Part print with two shaded views. Sizes in mm from the minimum x, y, z corner. Round coordinates to 2 decimals unless told otherwise and drop trailing zeros. Loops run counter-clockwise (first coordinate to the right, second up) from the corner with the lowest first, then second, coordinate; pieces in that order, holes last. Notation, with made-up numbers: M 18,-37 L 23,-37 A20 ccw 23,-25 Z; hole C 9,61.25 d10. An arc over 180 degrees is marked long. Answer as CSV lines item,"result". Start each with the question number.
Item 1: Wall check: line 1 (X direction, y = 7, z = 0.6) (1 decimal); line 2 (X direction, y = 1, z = 0.8) (1 decimal); line 3 (X direction, y = 10, z = 0.15) (1 decimal). Give the ranges that are in metal, low to high.
Item 2: Drop a flat-ended pin along its axis: pin 1 Ø0.7 at (y, z) = (11, 1) entering from -X. Give the stop position or say it passes through.
Item 3: Band-saw the part on A-A (z = 0.55). Give the cut face in (x, y) (1 decimal).
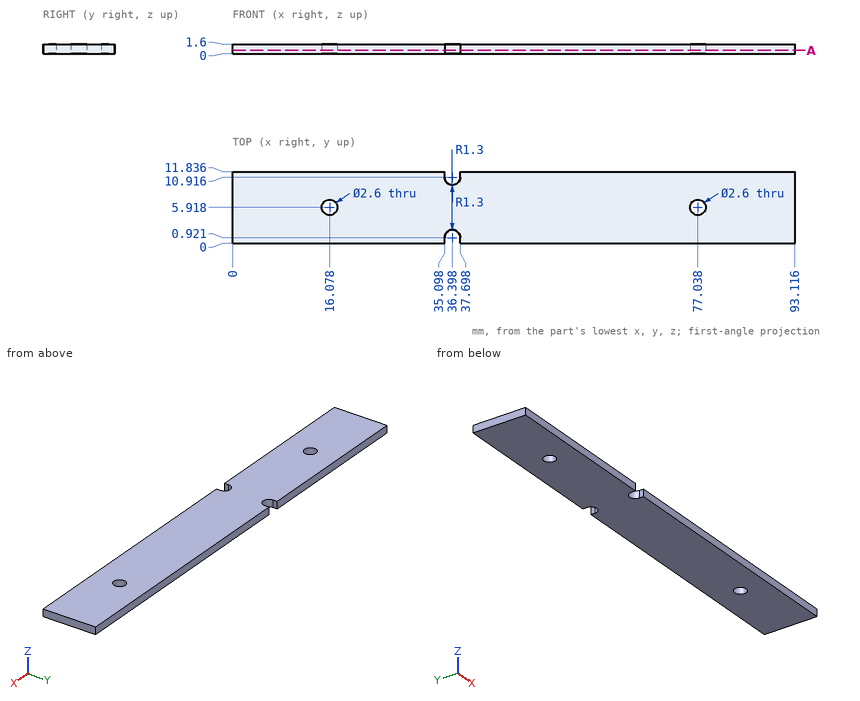
Answer block:
1,line 1,"x = 0 to 15.4, 16.8 to 76.3, 77.8 to 93.1"
1,line 2,"x = 0 to 35.1, 37.7 to 93.1"
1,line 3,"x = 0 to 35.5, 37.3 to 93.1"
2,pin 1,"stops at x = 0"
3,outline,"M 0,0 L 35.1,0 L 35.1,0.9 A1.3 cw 37.7,0.9 L 37.7,0 L 93.1,0 L 93.1,11.8 L 37.7,11.8 L 37.7,10.9 A1.3 cw 35.1,10.9 L 35.1,11.8 L 0,11.8 Z; hole C 16.1,5.9 d2.6; hole C 77,5.9 d2.6"
